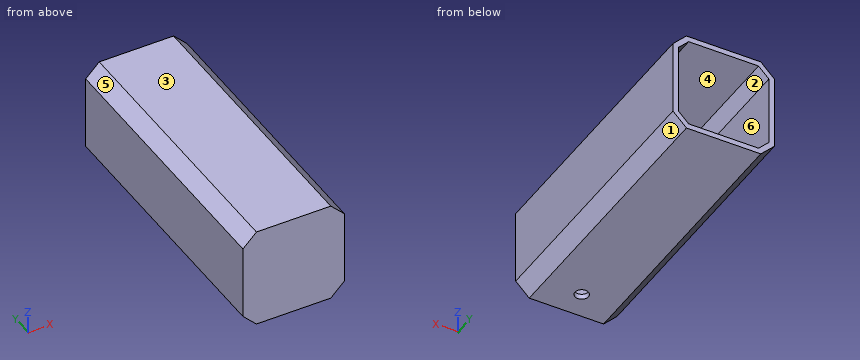
Autodesk Inventor part; units mm, degrees
ref_plane "YZ Plane" through (0, 0, 0) normal (1, 0, 0) x (0, 1, 0)
ref_plane "XZ Plane" through (0, 0, 0) normal (0, 1, 0) x (-1, 0, 0)
ref_plane "XY Plane" through (0, 0, 0) normal (0, 0, 1) x (1, 0, 0)
sketch "Sketch1" plane through (0, 0, 0) normal (0, 1, 0) x (-1, 0, 0)
  line L0 (65, 0) -> (10, 0)
  line L1 (0, -10) -> (0, -65)
  line L2 (10, -75) -> (65, -75)
  line L3 (75, -65) -> (75, -10)
  line L4 (75, -10) -> (65, 0)
  line L5 (10, 0) -> (0, -10)
  line L6 (0, -65) -> (10, -75)
  line L7 (75, -65) -> (65, -75)
  point P0 (0, 0)
  point P1 (75, 0)
  point P2 (0, -75)
  point P3 (0, 0)
  point P4 (75, -75)
  dimension "d0" = 75
  dimension "d1" = 75
  dimension "d2" = 10
  dimension "d3" = 10
  dimension "d4" = 10
  dimension "d5" = 10
  dimension "d6" = 10
  dimension "d7" = 10
  dimension "d8" = 10
  dimension "d9" = 10
extrude "Extrusion1" add sketch "Sketch1" along normal blind 5
sketch "Sketch2" plane through (0, 5, 0) normal (0, 1, 0) x (1, 0, 0)
  line L0 (-75, 10) -> (-65, 0)
  line L1 (-75, 65) -> (-75, 10)
  line L2 (-75, 10) -> (-75, 65)
  line L3 (-65, 75) -> (-75, 65)
  line L4 (-75, 65) -> (-65, 75)
  line L5 (-75, 10) -> (-65, 0)
  line L6 (-65, 0) -> (-10, 0)
  line L7 (-10, 0) -> (0, 10)
  line L8 (-10, 0) -> (0, 10)
  line L9 (0, 10) -> (0, 65)
  line L10 (0, 10) -> (0, 65)
  line L11 (0, 65) -> (-10, 75)
  line L12 (-10, 75) -> (-65, 75)
  line L13 (-10, 75) -> (-65, 75)
  line L14 (-65, 0) -> (-10, 0)
  line L15 (-11.6569, 71) -> (-4, 63.3431)
  line L16 (-4, 63.3431) -> (-4, 11.6569)
  line L17 (-4, 11.6569) -> (-11.6569, 4)
  line L18 (-11.6569, 4) -> (-63.3431, 4)
  line L19 (-63.3431, 4) -> (-71, 11.6569)
  line L20 (-71, 11.6569) -> (-71, 63.3431)
  line L21 (-71, 63.3431) -> (-63.3431, 71)
  line L22 (-63.3431, 71) -> (-11.6569, 71)
  point P0 (0, 0)
  dimension "d12" = 4
extrude "Extrusion2" add sketch "Sketch2" along normal blind 200
sketch "Sketch3" plane through (-10, 0, -75) normal (0, 0, -1) x (-1, 0, 0)
  circle A0 centre (27.5, 20) radius 5
  line L0 (0, 0) -> (0, 205) construction
  line L1 (55, 0) -> (0, 0) construction
  line L2 (0, 0) -> (55, 0) construction
  point P0 (-10, 0)
  point P1 (27.5, 0)
  dimension "d15" = 10
  dimension "d16" = 20
  dimension "d17" = 55
  dimension "d18" = 27.5
extrude "Extrusion3" cut sketch "Sketch3" against normal blind 4
sketch "Sketch4" plane through (0, 205, 0) normal (0, 1, 0) x (1, 0, 0)
  point P0 (0, 0)
properties part number "laser_leg"
Check sheet for the modelled part. Datum: model origin and axes. Units: mm. Face numbers are marked on the shaded views. A direction names the side the tool comes from. Round coordinates to 2 decimals unless told otherwise and drop trailing zeros. Loops run counter-clockwise (first coordinate to the right, second up) from the corner with the lowest first, then second, coordinate; pieces in that order, holes last. Notation, with made-up numbers: (8, 44) - (48, 44) arc R22 ccw to (48, 83) - close; hole circle Ø1 at (18, -33.75). An arc over 180 degrees is marked (long way). Write item = value, one per line. Start each with the question number.
Q1. Release check for a two-part mould opening along X. For the marked faces 1, 2, 3 and 4 record: pulls with the +X half, pulls with the -X half, needs draft (parallel to the pull), parting line crosses it, or undercut.
Q2. Access from +Z, -Z, +X, -X, +Y, -Y to the whole of each face (thin tool, end or side, straight path). Record for the marked faces 5 and 6.
Q3. Thickness scan on L1, parallel to Z at x = -61, y = 123; L2, parallel to Y at x = -37, z = -73. Record the ranges inside material, lowest first.
Q4. Section check B-B (y = 45). Record the boundary of the cut face in (x, z), plus the area to 3 significant figures.
Q5. Section check C-C (z = -23). Record the boundary of the cut face in (x, y).
Q6. Section check D-D (x = -24). Record the boundary of the cut face in (y, z).
Q7. Section check A-A (x = -37.5). Record the boundary of the cut face in (y, z).
Q8. Depth check by flat-ended pin: P1, Ø8, axis at x = -46, z = -51, coming from the +Y side. Enter the tip coordinate at first touch or a pass-through.
Derived:
q1.face_1 = pulls with the +X half
q1.face_2 = undercut
q1.face_3 = needs draft
q1.face_4 = undercut
q2.face_5 = +Z, -X, +Y, -Y
q2.face_6 = +Y
q3.L1 = -75 to -71, -4 to 0
q3.L2 = 0 to 15.03, 24.97 to 205
q4.outline = (-75, -65) - (-65, -75) - (-10, -75) - (0, -65) - (0, -10) - (-10, 0) - (-65, 0) - (-75, -10) - close; hole (-71, -63.34) - (-63.34, -71) - (-11.66, -71) - (-4, -63.34) - (-4, -11.66) - (-11.66, -4) - (-63.34, -4) - (-71, -11.66) - close
q4.area = 1,050 mm^2
q5.outline = (-75, 0) - (0, 0) - (0, 205) - (-4, 205) - (-4, 5) - (-71, 5) - (-71, 205) - (-75, 205) - close
q6.outline = (0, -75) - (205, -75) - (205, -71) - (5, -71) - (5, -4) - (205, -4) - (205, 0) - (0, 0) - close
q7.outline = (0, -75) - (15, -75) - (15, -71) - (5, -71) - (5, -4) - (205, -4) - (205, 0) - (0, 0) - close; (25, -75) - (205, -75) - (205, -71) - (25, -71) - close
q8.P1 = 5
